Verification items for the finished model (mm, model axes). Give positions to 0.01 mm unless a question says otherwise; leave off trailing zeros. Loops run counter-clockwise (first coordinate to the right, second up) from the corner with the lowest first, then second, coordinate; pieces in that order, holes last. Notation, with made-up numbers: M -4.75,5 L 44.25,5 A16 cw 44.25,14 Z; hole C -30.75,55 d4. An arc over 180 degrees is marked long. Answer in a Markdown table with one row per item.
Autodesk Inventor part; units mm, degrees
ref_plane "YZ Plane" through (0, 0, 0) normal (1, 0, 0) x (0, 1, 0)
ref_plane "XZ Plane" through (0, 0, 0) normal (0, 1, 0) x (-1, 0, 0)
ref_plane "XY Plane" through (0, 0, 0) normal (0, 0, 1) x (1, 0, 0)
sketch "Sketch1" plane through (0, 0, 0) normal (0, 1, 0) x (-1, 0, 0)
  line L0 (9, 21.5) -> (-9, 21.5)
  line L1 (-9, 21.5) -> (-9, -21.5)
  line L2 (-9, -21.5) -> (9, -21.5)
  line L3 (9, -21.5) -> (9, 21.5)
  line L4 (9, 21.5) -> (-9, -21.5) construction
  line L5 (-9, 21.5) -> (9, -21.5) construction
  point P0 (0, 0)
  dimension "d0" = 18
  dimension "d1" = 43
extrude "Extrusion1" add sketch "Sketch1" along normal blind 1.75
sketch "Sketch2" plane through (0, 1.75, 0) normal (0, 1, 0) x (1, 0, 0)
  circle A0 centre (-7.5, -17.5) radius 0.5
  line L0 (-9, -21.5) -> (9, -21.5)
  line L1 (-9, 21.5) -> (-9, -21.5)
  point P0 (0, 0)
  dimension "d4" = 1
  dimension "d5" = 4
  dimension "d6" = 1.5
extrude "Extrusion2" cut sketch "Sketch2" against normal blind 1.75
pattern_linear "Rectangular Pattern1" count 15 spacing 2.54 along (0, 0, -1) count 2 spacing 15 along (1, 0, 0) of "Extrusion2"
sketch "Sketch3" plane through (0, 0, 0) normal (0, -1, 0) x (1, 0, 0)
  circle A0 centre (0, 16.96) radius 0.5
  circle A1 centre (0, 19.5) radius 0.5
  circle A2 centre (2.54, 16.96) radius 0.5
  circle A3 centre (2.54, 19.5) radius 0.5
  line L0 (9, -21.5) -> (-9, -21.5)
  line L1 (-9, 21.5) -> (9, 21.5)
  circle A4 centre (-2.54, 19.5) radius 0.5
  circle A5 centre (-2.54, 16.96) radius 0.5
  point P0 (0, 0)
  dimension "d15" = 1
  dimension "d16" = 1
  dimension "d17" = 2.54
  dimension "d18" = 1
  dimension "d19" = 1
  dimension "d20" = 2.54
  dimension "d23" = 0
  dimension "d24" = 0
  dimension "d25" = 2.54
  dimension "d30" = 0
  dimension "d33" = 2
  dimension "d34" = 1
  dimension "d35" = 1
  dimension "d36" = 1.54
  dimension "d37" = 1.54
extrude "Extrusion3" cut sketch "Sketch3" against normal blind 10
properties part number "bord"
Item 1: Scan lines: L1, parallel to X at y = 1.45, z = -15.5; L2, parallel to Z at x = -2.54, y = 0.65; L3, parallel to X at y = 0.55, z = 9.5. Record each from-to range of solid material in increasing order. Write a range as [from, to].
Reported:
| item | result |
|---|---|
| L1 | x = [-9, -8], [-7, 7], [8, 9] |
| L2 | z = [-21.5, 16.46], [17.46, 19], [20, 21.5] |
| L3 | x = [-9, -7.82], [-7.18, 7.18], [7.82, 9] |
Item 2: Sectioned sample at A-A (x = 0). Record the cut outline in (y, z), and give its area (4 significant figures).
Reported:
| item | result |
|---|---|
| outline | M 0,-21.5 L 1.75,-21.5 L 1.75,16.46 L 0,16.46 Z; M 0,17.46 L 1.75,17.46 L 1.75,19 L 0,19 Z; M 0,20 L 1.75,20 L 1.75,21.5 L 0,21.5 Z |
| area | 71.75 mm^2 |
Item 3: Sectioned sample at C-C (z = -2.82). Record the cut outline in (x, y).
Reported:
| item | result |
|---|---|
| outline | M -9,0 L -8,0 L -8,1.75 L -9,1.75 Z; M -7,0 L 7,0 L 7,1.75 L -7,1.75 Z; M 8,0 L 9,0 L 9,1.75 L 8,1.75 Z |
Item 4: Sectioned sample at D-D (y = 0.45). State how many separate pieces and enclosed holes the cut face has, and give its area (3 significant figures).
Reported:
| item | result |
|---|---|
| separate pieces | 1 |
| enclosed holes | 36 |
| area | 746 mm^2 |
Item 5: Go/stop test with a flat-tipped pin: pin 1 (1 mm diameter, centred on x = 2, z = -10.5, fed in from -Y). Record where the tip stops, or that it passes through.
Reported:
| item | result |
|---|---|
| pin 1 | stops at y = 0 |
Item 6: Sectioned sample at B-B (z = 19.5). Record the cut outline in (x, y), and give its area (4 significant figures).
Reported:
| item | result |
|---|---|
| outline | M -9,0 L -3.04,0 L -3.04,1.75 L -9,1.75 Z; M -2.04,0 L -0.5,0 L -0.5,1.75 L -2.04,1.75 Z; M 0.5,0 L 2.04,0 L 2.04,1.75 L 0.5,1.75 Z; M 3.04,0 L 9,0 L 9,1.75 L 3.04,1.75 Z |
| area | 26.25 mm^2 |
Item 7: Release check for a two-part mould opening along X. For faces 1 (the flat face through (9, 1, 0)), 2 (the cylindrical face through (-7.23, 0.89, -18.48)), 3 (the cylindrical face through (7.962, 0.887, -2.628)) record: released by +X, released by -X, zero draft, split by the parting line, or undercut.
Reported:
| item | result |
|---|---|
| face 1 | released by +X |
| face 2 | undercut |
| face 3 | undercut |
